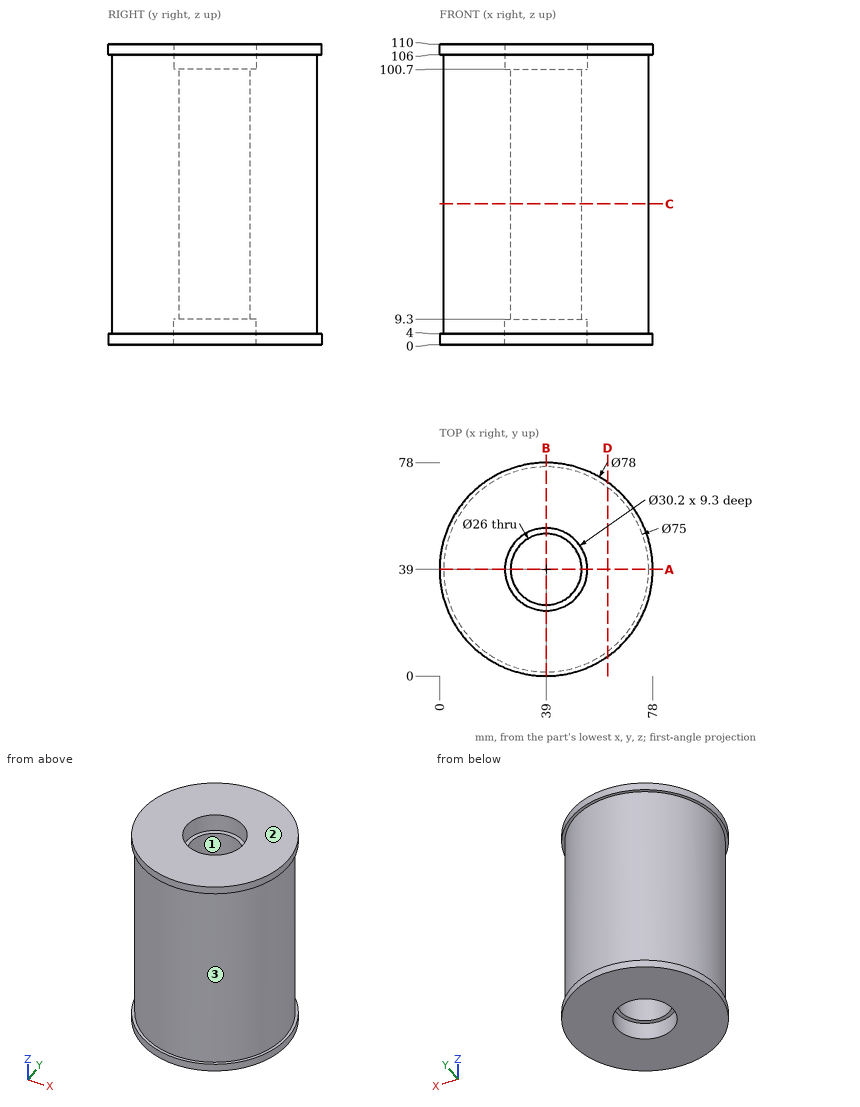
Could you check a few things on this drawing? It's one solid part, dimensions in mm from its lowest x, y, z. Coordinates: 2 decimals unless noted, no trailing zeros. Write each loop counter-clockwise with the first axis right and the second up, starting at its lowest first coordinate (ties: lowest second). Pieces come first, ordered by that corner, then holes. Notation, with made-up numbers: (50, 56) - (107, 56) arc R37 cw to (107, 93) - close; hole circle Ø11 at (18.25, 57.5). An arc over 180 degrees is marked (long way). Return JSON: item names as keys, results as strings. Group by question number.
Item 1: I'm going to push flat-ended pins straight in: pin 1 Ø1.5 at (y, z) = (46, 86.5) entering from +X; pin 2 Ø12 at (y, z) = (21.5, 30.5) entering from -X; pin 3 Ø1.5 at (x, z) = (23, 77.5) entering from +Y. Where does each tip first touch, or does it pass through?
Item 2: If we section it at C-C (z = 51.5): Write out the boundary of the cut face in (x, y), then the cut area to 3 significant figures.
Item 3: Please list where these lines run through material, in increasing order: probe 1 along Y at (x, z) = (39, 2.25); probe 2 along Y at (x, z) = (29, 40.5); probe 3 along Y at (x, z) = (72.5, 5).
Item 4: If we section it at D-D (x = 61.5): Write out the boundary of the cut face in (y, z), then the cut area to 3 significant figures.
Item 5: If we section it at A-A (y = 39): Write out the boundary of the cut face in (x, z), then the cut area to 3 significant figures.
Item 6: We'd pull the mould along Y, two halves only. Please class the marked faces 1, 2 and 3: pulls with the +Y half, pulls with the -Y half, needs draft (parallel to the pull), parting line crosses it, or undercut.
Return value:
{
 "1": {"pin 1": "stops at x = 75.98", "pin 2": "stops at x = 3.31", "pin 3": "stops at y = 73.26"},
 "2": {"outline": "circle Ø75 at (39, 39); hole circle Ø26 at (39, 39)", "area": "3,890 mm^2"},
 "3": {"probe 1": "y = 0 to 23.9, 54.1 to 78", "probe 2": "y = 2.86 to 30.69, 47.31 to 75.14", "probe 3": "y = 22.15 to 55.85"},
 "4": {"outline": "(7.14, 0) - (70.86, 0) - (70.86, 4) - (69, 4) - (69, 106) - (70.86, 106) - (70.86, 110) - (7.14, 110) - (7.14, 106) - (9, 106) - (9, 4) - (7.14, 4) - close", "area": "6,630 mm^2"},
 "5": {"outline": "(0, 0) - (23.9, 0) - (23.9, 9.3) - (26, 9.3) - (26, 100.7) - (23.9, 100.7) - (23.9, 110) - (0, 110) - (0, 106) - (1.5, 106) - (1.5, 4) - (0, 4) - close; (52, 9.3) - (54.1, 9.3) - (54.1, 0) - (78, 0) - (78, 4) - (76.5, 4) - (76.5, 106) - (78, 106) - (78, 110) - (54.1, 110) - (54.1, 100.7) - (52, 100.7) - close", "area": "5,340 mm^2"},
 "6": {"face 1": "undercut", "face 2": "needs draft", "face 3": "parting line crosses it"}
}
